Model file for the job. Use its own axes, mm. A direction names the side the tool comes from. Coordinates: 2 decimals unless noted, no trailing zeros. Loops run counter-clockwise (first coordinate to the right, second up) from the corner with the lowest first, then second, coordinate; pieces in that order, holes last. Notation, with made-up numbers: (-21.75, -11) -> (7.25, -11) arc R14 cw to (7.25, 0) -> close; hole circle Ø11 at (14, 41.25). An arc over 180 degrees is marked (long way). Use one line per item in the form item = value.
```python
from build123d import *

# Parameters (mm, degrees)
SKETCH2_W                    = 76.2
SKETCH2_H                    = 1.5875
BASE_FLANGE1_DEPTH           = 25.4
EDGE_FLANGE1_STRIP_W         = 16.51
EDGE_FLANGE1_STRIP_H         = 1.5875
EDGE_FLANGE1_STRIP_CUT_DEPTH = 76.2
EDGE_FLANGE1_DEPTH           = 76.2
FILLET1_R                    = 2.54
CUT_EXTRUDE1_DEPTH           = 104.382699985
SKETCH11_R                   = 1.5875
CUT_EXTRUDE2_DEPTH           = 105.014570043


# Sheet-metal steps are written as plain solids
with BuildPart() as part:
    # Sketch2 → Base-Flange1 (new body)
    with BuildSketch(Plane(origin=(0, 0, 0), x_dir=(1, 0, 0), z_dir=(0, 1, 0))):
        with Locations((38.1, -0.79375)):
            Rectangle(SKETCH2_W, SKETCH2_H)
    extrude(amount=BASE_FLANGE1_DEPTH)

    # Edge-Flange1 strip (across the edge) → Edge-Flange1 strip cut (cut)
    with BuildSketch(Plane(origin=(76.2, 25.4, 1.5875), x_dir=(0, -1, 0), z_dir=(-1, 0, 0))):
        with Locations((-1.5875, -0.79375)):
            Rectangle(EDGE_FLANGE1_STRIP_W, EDGE_FLANGE1_STRIP_H)
    extrude(amount=EDGE_FLANGE1_STRIP_CUT_DEPTH, mode=Mode.SUBTRACT)

    # Edge-Flange1 section (across the edge) → Edge-Flange1 (add)
    with BuildSketch(Plane(origin=(76.2, 25.4, 1.5875), x_dir=(0, -1, 0), z_dir=(-1, 0, 0))):
        with BuildLine():
            Line((0, 5.08), (0, 65.0875))
            Line((0, 65.0875), (1.5875, 65.0875))
            Line((1.5875, 65.0875), (1.5875, 5.08))
            ThreePointArc((1.5875, 5.08), (3.075397552, 1.487897552), (6.6675, 0))
            Line((6.6675, 0), (6.6675, -1.5875))
            ThreePointArc((6.6675, -1.5875), (1.952865536, 0.365365536), (0, 5.08))
        make_face()
    extrude(amount=EDGE_FLANGE1_DEPTH)

    # Fillet1
    fillet1_edges = [part.edges().sort_by_distance(p)[0] for p in [
        (76.2, 24.60625, 66.675),
        (0, 24.60625, 66.675),
        (0, 0, 0.79375),
        (76.2, 0, 0.79375),
    ]]
    fillet(fillet1_edges, radius=FILLET1_R)

    # Sketch10 → Cut-Extrude1 (cut, through all)
    with BuildSketch(Plane.XY.offset(1.5875)):
        with BuildLine():
            Line((7.3025, 11.67765), (8.5725, 11.67765))
            ThreePointArc((8.5725, 11.67765), (10.72515, 9.525), (8.5725, 7.37235))
            Line((8.5725, 7.37235), (7.3025, 7.37235))
            ThreePointArc((7.3025, 7.37235), (5.14985, 9.525), (7.3025, 11.67765))
        make_face()
        with BuildLine():
            Line((67.6275, 11.67765), (68.8975, 11.67765))
            ThreePointArc((68.8975, 11.67765), (71.05015, 9.525), (68.8975, 7.37235))
            Line((68.8975, 7.37235), (67.6275, 7.37235))
            ThreePointArc((67.6275, 7.37235), (65.47485, 9.525), (67.6275, 11.67765))
        make_face()
    extrude(amount=-CUT_EXTRUDE1_DEPTH, mode=Mode.SUBTRACT)

    # Sketch11 → Cut-Extrude2 (cut, through all)
    with BuildSketch(Plane.XZ.offset(-23.8125)):
        with Locations(Location((66.4972, 58.7502, 0), (0, 0, 270))):
            Circle(SKETCH11_R)
        with Locations(Location((66.4972, 23.8252, 0), (0, 0, 270))):
            Circle(SKETCH11_R)
        with Locations(Location((47.4472, 23.8252, 0), (0, 0, 270))):
            Circle(SKETCH11_R)
        with Locations(Location((47.4472, 58.7502, 0), (0, 0, 270))):
            Circle(SKETCH11_R)
    extrude(amount=-CUT_EXTRUDE2_DEPTH, mode=Mode.SUBTRACT)


solid = part.part
```
Q1. Band-saw the part on B-B, the plane x = 61. Write the cut outline in (y, z) (1 decimal).
Result:
outline = (0, 0) -> (18.7, 0) arc R6.7 ccw to (25.4, 6.7) -> (25.4, 66.7) -> (23.8, 66.7) -> (23.8, 6.7) arc R5.1 cw to (18.7, 1.6) -> (0, 1.6) -> close
Q2. Wall check: line 1 along Z through (x, y) = (11, 13); line 2 along Y through (x, z) = (59.5, 25.5); line 3 along Z through (x, y) = (6, 24.75) (3 decimals). Give the ranges that are in metal, low to high.
Result:
line_1 = 0 to 1.59
line_2 = 23.81 to 25.4
line_3 = 3.796 to 66.675
Q3. Band-saw the part on D-D, the plane y = 3.75. Write the cut outline in (x, z), and give its area (3 significant figures).
Result:
outline = (0, 0) -> (76.2, 0) -> (76.2, 1.59) -> (0, 1.59) -> close
area = 121 mm2
Q4. Pin check, flat tips, straight feed: pin 1 Ø1.5 at (x, y) = (13.5, 6) entering from +Z; pin 2 Ø1 at (x, z) = (68, 1) entering from +Y; pin 3 Ø5 at (y, z) = (21.5, 34.5) entering from -X; pin 4 Ø1.9 at (x, z) = (66.5, 58.75) entering from +Y. Stop position of each tip, or through.
Result:
pin_1 = 1.59
pin_2 = 22.95
pin_3 = 0
pin_4 = through
Q5. Mould opens along Z. For faces 4 (the face through (0.764, 24.595, 65.951)), 5 (the face through (38, 0, 1)), 6 (the face through (68.07, 24.6, 58.96)) say: released by +Z, released by -Z, zero draft, split by the parting line, or undercut.
Result:
face_4 = released by +Z
face_5 = zero draft
face_6 = undercut
Q6. Which spindle directions (+Z, -Z, +X, -X, +Y, -Y) get a long thin tool onto all of the face, cutting with end or side? Do faces 1 (the face through (38, 9, 1.588)), 2 (the face through (10.725, 9.572, 0.805)), 3 (the face through (0.724, 0.764, 0.783)). Say none if no direction does.
Result:
face_1 = +Z, +X, -X, -Y
face_2 = +Z, -Z
face_3 = +Z, -Z, -X, -Y
Q7. Band-saw the part on C-C, the plane z = 50. Write the cut outline in (x, y).
Result:
outline = (0, 23.81) -> (76.2, 23.81) -> (76.2, 25.4) -> (0, 25.4) -> close
Q8. Band-saw the part on A-A, the plane y = 9.75. Write the cut outline in (x, z).
Result:
outline = (0, 0) -> (5.16, 0) -> (5.16, 1.59) -> (0, 1.59) -> close; (10.71, 0) -> (65.49, 0) -> (65.49, 1.59) -> (10.71, 1.59) -> close; (71.04, 0) -> (76.2, 0) -> (76.2, 1.59) -> (71.04, 1.59) -> close
